Model file for the job. Use its own axes, mm. A direction names the side the tool comes from. Give positions to 0.01 mm unless a question says otherwise; leave off trailing zeros. Loops run counter-clockwise (first coordinate to the right, second up) from the corner with the lowest first, then second, coordinate; pieces in that order, holes last. Notation, with made-up numbers: M 26,33.25 L 85,33.25 A18 cw 85,48.25 Z; hole C -39,36.25 d10. An arc over 180 degrees is marked long. Answer in a Markdown table with one row per item.
```python
from build123d import *

# Parameters (mm, degrees)
BOSS_EXTRUDE1_DEPTH = 1.5875
BOSS_EXTRUDE2_DEPTH = 23.8125


with BuildPart() as part:
    # Sketch1 → Boss-Extrude1 (new body)
    with BuildSketch(Plane(origin=(0, 0, 0), x_dir=(1, 0, 0), z_dir=(0, 1, 0))):
        Polygon((0, 0), (15.362627366, 20.227448688), (-4.864821322, 35.590076054), (-20.227448688, 15.362627366), align=None)
    extrude(amount=BOSS_EXTRUDE1_DEPTH)

    # Sketch2 → Boss-Extrude2 (add)
    with BuildSketch(Plane(origin=(0, 1.5875, 0), x_dir=(1, 0, 0), z_dir=(0, 1, 0))):
        Polygon((-4.864821322, 35.590076054), (-5.824985532, 34.325860511), (14.402463156, 18.963233145), (15.362627366, 20.227448688), align=None)
    extrude(amount=BOSS_EXTRUDE2_DEPTH)


solid = part.part
```
Q1. Saw through at D-D (x = -12.5). Give the cut face in (y, z), and give its area (3 significant figures).
Reported:
| item | result |
|---|---|
| outline | M 0,-25.54 L 1.59,-25.54 L 1.59,-9.49 L 0,-9.49 Z |
| area | 25.5 mm² |
Q2. Saw through at A-A (z = -31). Give the cut face in (x, y), and give its area (3 significant figures).
Reported:
| item | result |
|---|---|
| outline | M -8.35,0 L 1.18,0 L 1.18,25.4 L -1.45,25.4 L -1.45,1.59 L -8.35,1.59 Z |
| area | 77.6 mm² |
Q3. Probe probe 1 along Y at (x, z) = (9, -14); probe 2 along X at (y, z) = (11, -22); probe 3 along Z at (x, y) = (-4.5, 20). List the from-to ranges inside material, lowest first.
Reported:
| item | result |
|---|---|
| probe 1 | 0 to 1.59 |
| probe 2 | 10.4 to 13.03 |
| probe 3 | -35.31 to -33.32 |
Q4. Saw through at B-B (x = 9). Give the cut face in (y, z).
Reported:
| item | result |
|---|---|
| outline | M 0,-25.06 L 25.4,-25.06 L 25.4,-23.07 L 1.59,-23.07 L 1.59,-11.85 L 0,-11.85 Z |
Q5. Saw through at C-C (y = 21.25). Give the cut face in (x, z), and give its area (3 significant figures).
Reported:
| item | result |
|---|---|
| outline | M -5.82,-34.33 L -4.86,-35.59 L 15.36,-20.23 L 14.4,-18.96 Z |
| area | 40.3 mm² |
Q6. 3-axis set-ups, long thin cutter, end or side, ignore diameter. For faces 1 (the face through (4.15, 13.33, -26.75)), 2 (the face through (5.39, 12.52, -27.8)): which of +Z, -Z, +X, -X, +Y, -Y reach the whole face in a straight line?
Reported:
| item | result |
|---|---|
| face 1 | +Z, -X, +Y |
| face 2 | -Z, +X, +Y, -Y |
Q7. Drop flat-ended pins along their axis: pin 1 (10.5 mm diameter, centred on x = -3.5, z = -23.5, fed in from +Y); pin 2 (1.5 mm diameter, centred on y = 5, z = -31, fed in from -X); pin 3 (10 mm diameter, centred on x = 2.5, y = 15, fed in from -Z). Give the stop position or say it passes through.
Reported:
| item | result |
|---|---|
| pin 1 | y = 1.59 |
| pin 2 | x = -2.43 |
| pin 3 | z = -33.79 |
